The model under review builds one solid part; all positions refer to its coordinate system, in mm. A direction names the side the tool comes from. Round coordinates to 2 decimals unless told otherwise and drop trailing zeros. Write each loop counter-clockwise with the first axis right and the second up, starting at its lowest first coordinate (ties: lowest second). Pieces come first, ordered by that corner, then holes. Notation, with made-up numbers: (75, -35.5) - (120, -35.5) arc R14 cw to (120, -17.5) - close; hole circle Ø5 at (89, 33.5). An arc over 180 degrees is marked (long way). Return JSON: item names as keys, results as strings.
from build123d import *

# Parameters (mm, degrees)
F0_R          = 9.398
F2_DEPTH      = 17.78
F3_DEPTH      = 14.478
F1_W          = 12.7
F1_H          = 12.7
F4_DEPTH      = 107
F4_DEPTH_BACK = 17.781
F5_D          = 5.1308
F6_R          = 2.54
F7_R          = 2.54
F8_R          = 2.54
F9_R          = 5.08
F10_DEPTH     = 6.35


# Not quite as in the source:
# - an extrude ends at something that could not be found from the text; its depth is read off the source's solid


with BuildPart() as f2:
    # F0 (on Top) → F2 (new body)
    with BuildSketch(Plane.XY):
        with BuildLine():
            ThreePointArc((10.9985226281, 32.7464543073), (0, 39.0964543073), (-10.9985226281, 32.7464543073))
            Line((-10.9985226281, 32.7464543073), (-33.8585226281, -6.8482271537))
            ThreePointArc((-33.8585226281, -6.8482271537), (-33.8585226281, -19.5482271537), (-22.86, -25.8982271537))
            Line((-22.86, -25.8982271537), (22.86, -25.8982271537))
            ThreePointArc((22.86, -25.8982271537), (33.8585226281, -19.5482271537), (33.8585226281, -6.8482271537))
            Line((33.8585226281, -6.8482271537), (10.9985226281, 32.7464543073))
        make_face()
        with Locations((-22.86, -13.1982271537)):
            Circle(F0_R, mode=Mode.SUBTRACT)
        with Locations((22.86, -13.1982271537)):
            Circle(F0_R, mode=Mode.SUBTRACT)
        with Locations((0, 26.3964543073)):
            Circle(F0_R, mode=Mode.SUBTRACT)
    extrude(amount=F2_DEPTH)

    # F0 (on Top) → F3 (join)
    with BuildSketch(Plane.XY):
        with Locations((-22.86, -13.1982271537)):
            Circle(F0_R)
        with Locations((22.86, -13.1982271537)):
            Circle(F0_R)
        with Locations((0, 26.3964543073)):
            Circle(F0_R)
    extrude(amount=F3_DEPTH)

    # F1 (on face) → F4 (cut, two sides)
    with BuildSketch(Plane.XY) as f4_sk:
        Rectangle(F1_W, F1_H)
    extrude(amount=-F4_DEPTH, mode=Mode.SUBTRACT)
    extrude(f4_sk.sketch, amount=F4_DEPTH_BACK, mode=Mode.SUBTRACT)

    # F5 (through all)
    with Locations(Plane(origin=(0, 0, 0), x_dir=(1, 0, 0), z_dir=(0, 0, -1))):
        with Locations((-22.86, 13.1982271537), (22.86, 13.1982271537), (0, -26.3964543073)):
            Hole(F5_D / 2)

    # F6
    f6_edges = [f2.edges().sort_by_distance(p)[0] for p in [
        (-22.428523, 12.949114, 17.78),
    ]]
    fillet(f6_edges, radius=F6_R)

    # F7
    f7_edges = [f2.edges().sort_by_distance(p)[0] for p in [
        (22.428523, 12.949114, 0),
    ]]
    fillet(f7_edges, radius=F7_R)

    # F8
    f8_edges = [f2.edges().sort_by_distance(p)[0] for p in [
        (6.35, 0, 0),
        (0, -6.35, 0),
        (0, 6.35, 0),
        (-6.35, 0, 0),
    ]]
    fillet(f8_edges, radius=F8_R)

    # F9 (on face) → F10 (cut)
    with BuildSketch(Plane.XY):
        with Locations((22.86, -13.1982271537)):
            Circle(F9_R)
        with Locations((0, 26.3964543073)):
            Circle(F9_R)
        with Locations((-22.86, -13.1982271537)):
            Circle(F9_R)
    extrude(amount=F10_DEPTH, mode=Mode.SUBTRACT)


solid = f2.part
(1) Add section A-A (x = 0). Write out the cut boundary in (y, z), plus the area to 3 significant figures.
Filled in:
{"outline": "(-25.9, 2.54) arc R2.54 ccw to (-23.36, 0) - (-8.89, 0) arc R2.54 ccw to (-6.35, 2.54) - (-6.35, 17.78) - (-23.36, 17.78) arc R2.54 ccw to (-25.9, 15.24) - close; (6.35, 2.54) arc R2.54 ccw to (8.89, 0) - (21.32, 0) - (21.32, 6.35) - (23.83, 6.35) - (23.83, 14.48) - (17, 14.48) - (17, 17.78) - (6.35, 17.78) - close; (28.96, 6.35) - (31.48, 6.35) - (31.48, 0) - (36.56, 0) arc R2.54 ccw to (39.1, 2.54) - (39.1, 15.24) arc R2.54 ccw to (36.56, 17.78) - (35.79, 17.78) - (35.79, 14.48) - (28.96, 14.48) - close", "area": "753 mm2"}
(2) Wall thickness on line 1 (X direction, y = -17, z = 15); line 2 (X direction, y = 21, z = 2.5); line 3 (Z direction, x = 0, y = 35.5): over which ranges is each line inside the solid? List them lowest first.
Filled in:
{"line 1": "x = -34.98 to -31.45, -14.27 to 14.27, 31.45 to 34.98", "line 2": "x = -17.78 to 17.78", "line 3": "z = 0 to 14.48"}
(3) Add section B-B (z = 3.75). Write out the cut boundary in (x, y), plus the area to 3 significant figures.
Filled in:
{"outline": "(-33.86, -6.85) arc R12.7 ccw to (-22.86, -25.9) - (22.86, -25.9) arc R12.7 ccw to (33.86, -6.85) - (11, 32.75) arc R12.7 ccw to (-11, 32.75) - close; hole circle Ø10.16 at (-22.86, -13.2); hole (-6.35, -6.35) - (6.35, -6.35) - (6.35, 6.35) - (-6.35, 6.35) - close; hole circle Ø10.16 at (0, 26.4); hole circle Ø10.16 at (22.86, -13.2)", "area": "2,750 mm2"}
(4) Add section C-C (z = 11.75). Write out the cut boundary in (x, y), plus the area to 3 significant figures.
Filled in:
{"outline": "(-33.86, -6.85) arc R12.7 ccw to (-22.86, -25.9) - (22.86, -25.9) arc R12.7 ccw to (33.86, -6.85) - (11, 32.75) arc R12.7 ccw to (-11, 32.75) - close; hole circle Ø5.13 at (-22.86, -13.2); hole (-6.35, -6.35) - (6.35, -6.35) - (6.35, 6.35) - (-6.35, 6.35) - close; hole circle Ø5.13 at (0, 26.4); hole circle Ø5.13 at (22.86, -13.2)", "area": "2,930 mm2"}
(5) Clearance check with flat-ended pins moving along their axes: pin 1 Ø10 at (y, z) = (-15, 2.5) entering from +X; pin 2 Ø10 at (x, y) = (18, 31) entering from +Z; pin 3 Ø1 at (y, z) = (18, 2) entering from -X; pin 4 Ø6 at (x, y) = (22.86, -13.2) entering from -Z. State where each tip first meets the part, or that it passes through.
Filled in:
{"pin 1": "stops at x = 35.56", "pin 2": "passes through", "pin 3": "stops at x = -19.75", "pin 4": "stops at z = 6.35"}
(6) For faces 1 (the cylindrical face through (-23.961, -18.157, 3.131)), 2 (the flat face through (6.35, 0, 10)), 3 (the cylindrical face through (0.32, -25.17, 17.02)), list the 3-axis set-ups (+Z, -Z, +X, -X, +Y, -Y) from which the entire face can be reached by the end or side of a thin tool; tool diameter is ignored.
Filled in:
{"face 1": "-Z", "face 2": "+Z, -Z", "face 3": "+Z, +X, -X, -Y"}
(7) Mouldability with a two-part tool opening along Y and no side actions: class faces 4 (the flat face through (0, -25.898, 9)), 5 (the flat face through (-22.269, 13.226, 8.801)), 6 (the cylindrical face through (15.93, -6.85, 16.11)) as released by +Y, released by -Y, zero draft, split by the parting line, or undercut.
Filled in:
{"face 4": "released by -Y", "face 5": "released by +Y", "face 6": "undercut"}
